Build history of the part. All positions in model axes, mm. A direction names the side the tool comes from. Round coordinates to 2 decimals unless told otherwise and drop trailing zeros. Loops run counter-clockwise (first coordinate to the right, second up) from the corner with the lowest first, then second, coordinate; pieces in that order, holes last. Notation, with made-up numbers: (25, -4) - (44, -4) arc R28 cw to (44, 30) - close; hole circle Ø5 at (51.25, 25). An arc over 180 degrees is marked (long way). Answer as CSV lines item,"result". Start each with the question number.
```python
from build123d import *

# Parameters (mm, degrees)
F0_R     = 101.6
F0_R_2   = 96.8375
F1_DEPTH = 152.4
F4_DEPTH = 12.7


with BuildPart() as f1:
    # F0 (on Top) → F1 (new body)
    with BuildSketch(Plane.XY):
        Circle(F0_R)
        Circle(F0_R_2, mode=Mode.SUBTRACT)
    extrude(amount=F1_DEPTH)

    # F2 (on Right) → F3 (revolve)
    with BuildSketch(Plane.YZ):
        with BuildLine():
            Line((-101.6, 152.4), (-96.8375, 152.4))
            ThreePointArc((-96.8375, 152.4), (-93.8204640896, 162.6881758587), (-85.725, 169.717580482))
            ThreePointArc((-85.725, 169.717580482), (-82.8148388415, 170.774666369), (-79.771875, 171.3463652414))
            Line((-79.771875, 171.3463652414), (-79.771875, 174.8506403027))
            Line((-79.771875, 174.8506403027), (-81.75625, 174.8506403027))
            Line((-81.75625, 174.8506403027), (-85.725, 174.8506403027))
            ThreePointArc((-85.725, 174.8506403027), (-97.2303248333, 166.1481532851), (-101.6, 152.4))
        make_face()
    revolve(axis=Axis((0, 0, 76.2), (0, 0, 1)))

    # F4 (add): a face of the model
    f4_faces = [f1.faces().sort_by_distance(p)[0] for p in [
        (0, 82.1965441527, 174.8506403027),
    ]]
    extrude(f4_faces, amount=F4_DEPTH)

    # F5 (on Right) → F6 (revolve)
    with BuildSketch(Plane.YZ):
        with BuildLine():
            Line((0, -22.4506403027), (0, -19.05))
            Line((0, -19.05), (-77.7875, -19.05))
            ThreePointArc((-77.7875, -19.05), (-81.8496787146, -18.6118565461), (-85.725, -17.317580482))
            ThreePointArc((-85.725, -17.317580482), (-93.8204640896, -10.2881758587), (-96.8375, 0))
            Line((-96.8375, 0), (-101.6, 0))
            ThreePointArc((-101.6, 0), (-97.2303248333, -13.7481532851), (-85.725, -22.4506403027))
            Line((-85.725, -22.4506403027), (-77.7875, -22.4506403027))
            Line((-77.7875, -22.4506403027), (0, -22.4506403027))
        make_face()
    revolve(axis=Axis((0, 0, -11.2253201513), (0, 0, 1)))


solid = f1.part
```
Q1. Wall check: probe 1 along X at (y, z) = (0, 31); probe 2 along X at (y, z) = (0, 175.5) (3 decimals); probe 3 along Z at (x, y) = (-24, -40). Give the ranges that are in metal, low to high. Write a range as [from, to].
Q2. Band-saw the part on A-A, the plane z = 30.5. List the corners of the cut face in (x, y) (1 decimal).
Q3. Tool access for faces 4 (the flat face through (-76, 25, 187.551)), 5 (the flat face through (1, -1, -19.05)), 6 (the cylindrical face through (-20.992, -94.535, 75.133)): list every direction of +Z, -Z, +X, -X, +Y, -Y with a clear straight run to the whole face (end or side of a thin tool).
Q4. Two-plate mould, pull along Y, no slides. Class faces 1 (the cylindrical face through (72.28, -46.09, 181.11)), 2 (the flat face through (1, 1, -22.451)), 3 (the cylindrical face through (23.96, -76.09, 179.34)): released by +Y, released by -Y, zero draft, split by the parting line, or undercut.
Q5. Pin check, flat tips, straight feed: pin 1 Ø1 at (x, y) = (-46, 50.5) entering from +Z; pin 2 Ø3 at (x, z) = (41, 33) entering from +Y; pin 3 Ø8 at (x, z) = (-42, 108.5) entering from +Y. Stop position of each tip, or through.
Reported:
1,probe 1,"x = [-101.6, -96.84], [96.84, 101.6]"
1,probe 2,"x = [-85.725, -79.772], [79.772, 85.725]"
1,probe 3,"z = [-22.45, -19.05]"
2,outline,"circle Ø203.2 at (0, 0); hole circle Ø193.7 at (0, 0)"
3,face 4,"+Z, +X, -X, +Y, -Y"
3,face 5,"+Z"
3,face 6,"none"
4,face 1,"split by the parting line"
4,face 2,"zero draft"
4,face 3,"undercut"
5,pin 1,"stops at z = -19.05"
5,pin 2,"stops at y = 93.61"
5,pin 3,"stops at y = 94.23"
